Input: dimensioned drawing with shaded views. Units: mm. Origin: part minimum x, y, z. Round coordinates to 2 decimals unless told otherwise and drop trailing zeros. Write each loop counter-clockwise with the first axis right and the second up, starting at its lowest first coordinate (ties: lowest second). Pieces come first, ordered by that corner, then holes. Notation, with made-up numbers: M -28,80.25 L 11,80.25 A12 cw 11,84.25 Z; hole C 32.25,2.25 d7. An arc over 180 degrees is marked long. Answer in a Markdown table with one row per item. Add a question column.
Item 1: Cut plane B-B on y = 1.5. Return loops of the section in (x, z), and give its area (3 significant figures).
Item 2: Contact query for a flat-ended pin moving along its axis: pin 1 (1 mm diameter, centred on x = 1.5, y = 2.5, fed in from -Z). Output: stop coordinate, or through.
Item 3: Cut plane A-A on z = 0.4. Return loops of the section in (x, y).
Item 4: Cut plane C-C on x = 5.25. Return loops of the section in (y, z), and give its area (3 significant figures).
Item 5: Material intervals for probe 1 along Y at (x, z) = (1.5, 0.1); probe 2 along Y at (x, z) = (7.75, 0.1); probe 3 along X at (y, z) = (6.5, 0.25), sorted ascending.
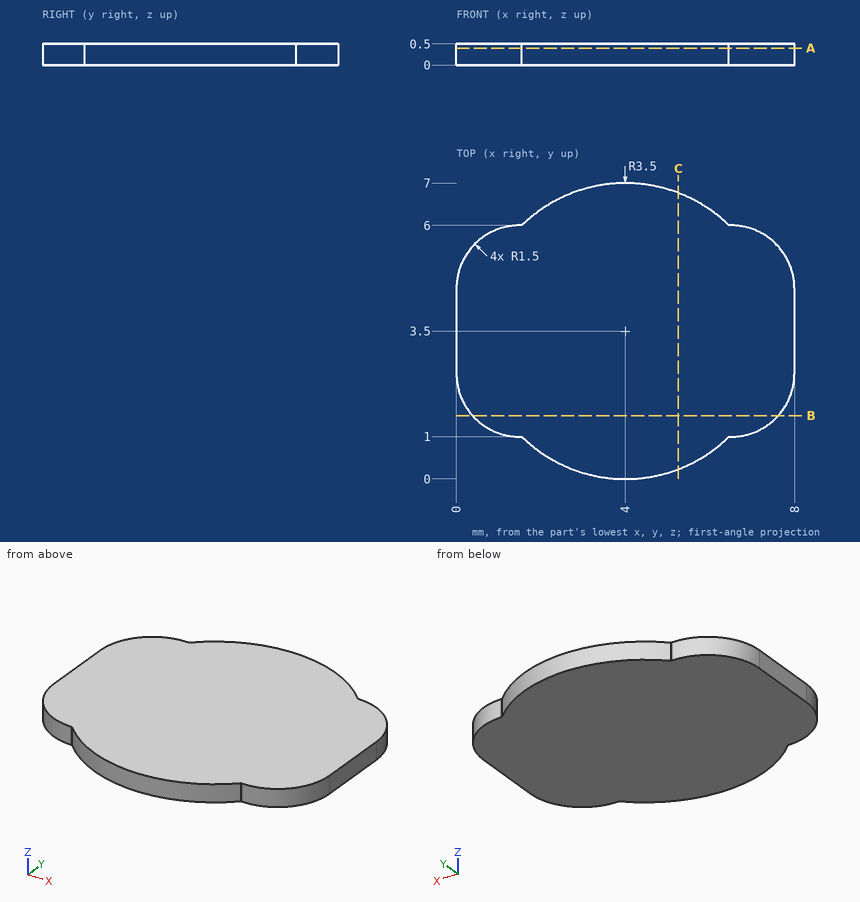
Results below:
| question | item | result |
|---|---|---|
| 1 | outline | M 0.38,0 L 7.62,0 L 7.62,0.5 L 0.38,0.5 Z |
| 1 | area | 3.62 mm2 |
| 2 | pin 1 | z = 0 |
| 3 | outline | M 0,2.5 A1.5 ccw 1.5,1 L 1.55,1 A3.5 ccw 6.45,1 L 6.5,1 A1.5 ccw 8,2.5 L 8,4.5 A1.5 ccw 6.5,6 L 6.45,6 A3.5 ccw 1.55,6 L 1.5,6 A1.5 ccw 0,4.5 Z |
| 4 | outline | M 0.23,0 L 6.77,0 L 6.77,0.5 L 0.23,0.5 Z |
| 4 | area | 3.27 mm2 |
| 5 | probe 1 | 1 to 6 |
| 5 | probe 2 | 1.67 to 5.33 |
| 5 | probe 3 | 2.2 to 5.8 |
